Build history of the part. All positions in model axes, mm. A direction names the side the tool comes from. Round coordinates to 2 decimals unless told otherwise and drop trailing zeros. Order: outer loops, then holes, each group sorted by start corner. A loop starts at its lowest first (then second) coordinate and runs counter-clockwise, first axis right, second up. Notation, with made-up numbers: (30, 8) -> (76, 8) arc R25 ccw to (76, 26) -> close; hole circle Ø8 at (-5.5, 64.25). An arc over 180 degrees is marked (long way). Use a Markdown table: item, result. Add a question column.
Item 1: Slice it at C-C, the plane y = 4. Give the cut face in (x, z), plus the area to 3 significant figures.
Item 2: Pin check, flat tips, straight feed: pin 1 (5.5 mm diameter, centred on x = 9.8, z = -9.71, fed in from -Y); pin 2 (2.5 mm diameter, centred on x = 32, z = -21.5, fed in from +Y). Stop position of each tip, or through.
Item 3: Two-plate mould, pull along X, no slides. Class faces 1 (the face through (24, 0, -14)), 2 (the face through (16, 14, -23)), 3 (the face through (0, 9, -17)): released by +X, released by -X, zero draft, split by the parting line, or undercut.
Item 4: 3-axis set-ups, long thin cutter, end or side, ignore diameter. For faces 4 (the face through (6.26, 11.483, -27.968)), 5 (the face through (12.33, 9.63, -8.1)), 6 (the face through (16, 9, -22)): which of +Z, -Z, +X, -X, +Y, -Y reach the whole face in a straight line?
Item 5: Slice it at D-D, the plane y = 10.5. Give the cut face in (x, z).
Item 6: Slice it at B-B, the plane z = -9.71. Give the cut face in (x, y), plus the area to 3 significant figures.
Item 7: Probe L1, parallel to X at y = 8.25, z = -9.71; L2, parallel to X at y = 9.75, z = -18.5; L3, parallel to Z at x = 7.5, y = 5.75. List the from-to ranges inside material, lowest first.
Item 8: Slice it at A-A, the plane x = 9.8. Give the cut face in (y, z), plus the area to 3 significant figures.
from build123d import *

# Parameters (mm, degrees)
ESBO_O1_W                = 48
ESBO_O1_H                = 35
RESSALTO_EXTRUS_O1_DEPTH = 19
ESBO_O4_R                = 5.1
CORTE_EXTRUS_O3_DEPTH    = 25
ESBO_O7_R                = 3
CORTE_EXTRUS_O7_DEPTH    = 63.369864518
ESBO_O8_R                = 3
CORTE_EXTRUS_O8_DEPTH    = 63.369864518
ESBO_O9_R                = 2
CORTE_EXTRUS_O9_DEPTH    = 17
ESBO_O6_R                = 1.5
CORTE_EXTRUS_O10_DEPTH   = 10


with BuildPart() as part:
    # Esboço1 → Ressalto-extrusão1 (new body)
    with BuildSketch(Plane(origin=(0, 0, 0), x_dir=(1, 0, 0), z_dir=(0, 1, 0))):
        with Locations((24, 17.5)):
            Rectangle(ESBO_O1_W, ESBO_O1_H)
    extrude(amount=RESSALTO_EXTRUS_O1_DEPTH)

    # Esboço4 → Corte-extrusão3 (cut)
    with BuildSketch(Plane(origin=(0, 19, 0), x_dir=(1, 0, 0), z_dir=(0, 1, 0))):
        with Locations(Location((24, 21.5, 0), (0, 0, 270))):
            Circle(ESBO_O4_R)
    extrude(amount=-CORTE_EXTRUS_O3_DEPTH, mode=Mode.SUBTRACT)

    # Esboço7 → Corte-extrusão7 (cut, through all)
    with BuildSketch(Plane(origin=(0, 19, 0), x_dir=(1, 0, 0), z_dir=(0, 1, 0))):
        with Locations(Location((9.8, 9.71, 0), (0, 0, 270))):
            Circle(ESBO_O7_R)
        with Locations(Location((38.2, 9.71, 0), (0, 0, 270))):
            Circle(ESBO_O7_R)
    extrude(amount=-CORTE_EXTRUS_O7_DEPTH, mode=Mode.SUBTRACT)

    # Esboço8 → Corte-extrusão8 (cut, through all)
    with BuildSketch(Plane.XZ):
        with Locations(Location((6, -18.5, 0), (0, 0, 270))):
            Circle(ESBO_O8_R)
    extrude(amount=-CORTE_EXTRUS_O8_DEPTH, mode=Mode.SUBTRACT)

    # Esboço9 → Corte-extrusão9 (cut)
    with BuildSketch(Plane(origin=(0, 0, -35), x_dir=(-1, 0, 0), z_dir=(0, 0, -1))):
        with Locations((-6, 9.5)):
            Circle(ESBO_O9_R)
    extrude(amount=-CORTE_EXTRUS_O9_DEPTH, mode=Mode.SUBTRACT)

    # Esboço6 → Corte-extrusão10 (cut)
    with BuildSketch(Plane(origin=(0, 19, 0), x_dir=(1, 0, 0), z_dir=(0, 1, 0))):
        with Locations(Location((23.767635295, 29.496624703, 0), (0, 0, 270))):
            Circle(ESBO_O6_R)
        with Locations(Location((16, 21.5, 0), (0, 0, 270))):
            Circle(ESBO_O6_R)
        with Locations(Location((32, 21.5, 0), (0, 0, 270))):
            Circle(ESBO_O6_R)
        with Locations(Location((23.767635295, 13.503375297, 0), (0, 0, 270))):
            Circle(ESBO_O6_R)
    extrude(amount=-CORTE_EXTRUS_O10_DEPTH, mode=Mode.SUBTRACT)


solid = part.part
Check sheet entries:
| question | item | result |
|---|---|---|
| 1 | outline | (0, -35) -> (48, -35) -> (48, 0) -> (0, 0) -> close; hole circle Ø6 at (6, -18.5); hole circle Ø6 at (9.8, -9.71); hole circle Ø10.2 at (24, -21.5); hole circle Ø6 at (38.2, -9.71) |
| 1 | area | 1,510 mm2 |
| 2 | pin 1 | through |
| 2 | pin 2 | y = 9 |
| 3 | face 1 | zero draft |
| 3 | face 2 | undercut |
| 3 | face 3 | released by -X |
| 4 | face 4 | -Z |
| 4 | face 5 | +Y, -Y |
| 4 | face 6 | +Y |
| 5 | outline | (0, -35) -> (4.27, -35) -> (4.27, -20.95) arc R3 cw (long way) to (7.73, -20.95) -> (7.73, -35) -> (48, -35) -> (48, 0) -> (0, 0) -> close; hole circle Ø6 at (9.8, -9.71); hole circle Ø3 at (16, -21.5); hole circle Ø10.2 at (24, -21.5); hole circle Ø3 at (23.77, -29.5); hole circle Ø3 at (23.77, -13.5); hole circle Ø3 at (32, -21.5); hole circle Ø6 at (38.2, -9.71) |
| 6 | outline | (0, 0) -> (6.8, 0) -> (6.8, 19) -> (0, 19) -> close; (12.8, 0) -> (35.2, 0) -> (35.2, 19) -> (12.8, 19) -> close; (41.2, 0) -> (48, 0) -> (48, 19) -> (41.2, 19) -> close |
| 6 | area | 684 mm2 |
| 7 | L1 | 0 to 6.8, 12.8 to 35.2, 41.2 to 48 |
| 7 | L2 | 0 to 3, 9 to 19.88, 28.12 to 48 |
| 7 | L3 | -35 to -21.1, -15.9 to -11.64, -7.78 to 0 |
| 8 | outline | (0, -35) -> (19, -35) -> (19, -12.71) -> (0, -12.71) -> close; (0, -6.71) -> (19, -6.71) -> (19, 0) -> (0, 0) -> close |
| 8 | area | 551 mm2 |
